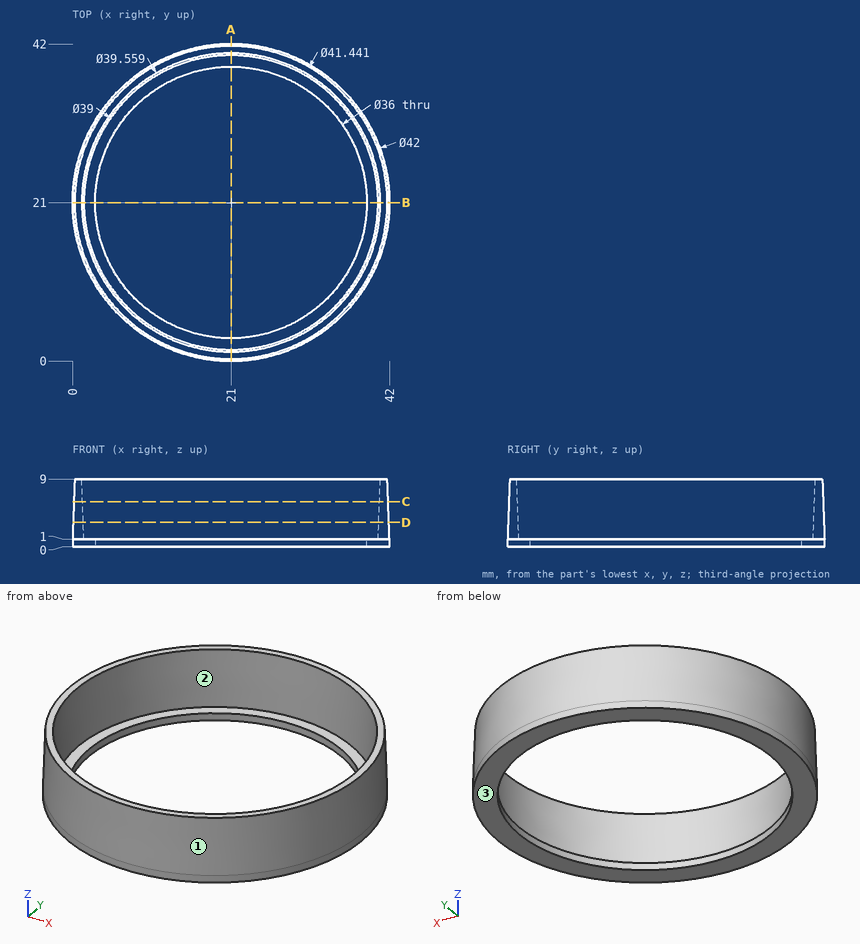
The figure shows three views and two pictorial views of one solid part (mm, origin at its lowest corner). Answer the questions. Coordinates: 2 decimals unless noted, no trailing zeros. Loops run counter-clockwise (first coordinate to the right, second up) from the corner with the lowest first, then second, coordinate; pieces in that order, holes last.
1) Flat-ended cylindrical pins translate along their axes: pin 1 Ø2 at (y, z) = (23.5, 7) entering from +X; pin 2 Ø1 at (x, z) = (10.5, 6.5) entering from +Y; pin 3 Ø3 at (x, z) = (17, 2.5) entering from +Y (1 decimal). Find the tip coordinate at first contact, or state that the pin passes through.
2) Find the intervals of material crossed by L1, parallel to Y at x = 21, z = 0.45; L2, parallel to Y at x = 4.5, z = 8.5 (1 decimal); L3, parallel to Z at x = 9, y = 34.5, in increasing order.
3) Find section D-D on z = 3.25. Write down the section's boundary in (x, y), then the cut area to 3 significant figures.
4) Find section C-C on z = 6. Write down the section's boundary in (x, y) (1 decimal).
5) Determine the mould class of the marked faces 1, 2 and 3 for opening direction Y: pulls with the +Y half, pulls with the -Y half, needs draft (parallel to the pull), parting line crosses it, or undercut.
6) Find section A-A on x = 21. Write down the section's boundary in (y, z).
Values:
1. pin 1: stops at x = 41.74
1. pin 2: stops at y = 39.25
1. pin 3: stops at y = 41.8
2. L1: y = 0 to 3, 39 to 42
2. L2: y = 8.4 to 10.1, 31.9 to 33.6
2. L3: z = 0 to 1
3. outline: circle Ø41.84 at (21, 21); hole circle Ø39.16 at (21, 21)
3. area: 171 mm2
4. outline: circle Ø41.7 at (21, 21); hole circle Ø39.3 at (21, 21)
5. face 1: parting line crosses it
5. face 2: undercut
5. face 3: needs draft
6. outline: (0, 0) - (3, 0) - (3, 1) - (1.5, 1) - (1.22, 9) - (0.28, 9) - (0, 1) - close; (39, 0) - (42, 0) - (42, 1) - (41.72, 9) - (40.78, 9) - (40.5, 1) - (39, 1) - close
